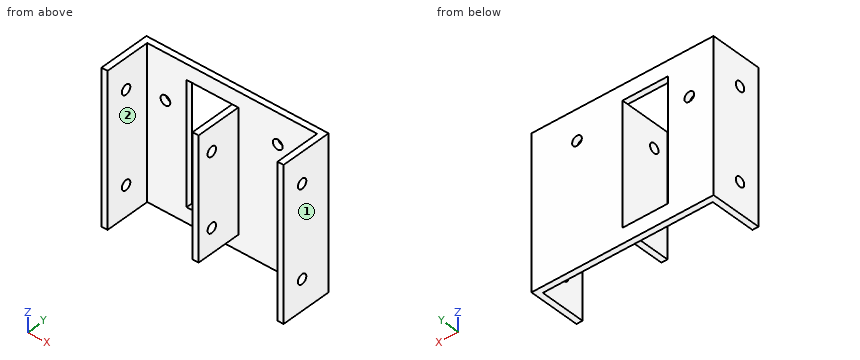
from build123d import *

# Parameters (mm, degrees)
BOSS_EXTRUDE1_DEPTH = 50
SKETCH2_R           = 1.6
CUT_EXTRUDE1_DEPTH  = 80.931220434
SKETCH3_W           = 2
SKETCH3_H           = 40
BOSS_EXTRUDE2_DEPTH = 17
SKETCH5_R           = 1.6
CUT_EXTRUDE3_DEPTH  = 2
SKETCH6_R           = 1.6
CUT_EXTRUDE4_DEPTH  = 80.931220434
SKETCH7_W           = 15
SKETCH7_H           = 40
CUT_EXTRUDE5_DEPTH  = 2


with BuildPart() as part:
    # Sketch1 → Boss-Extrude1 (new body)
    with BuildSketch(Plane.XY):
        Polygon((0, 0), (0, 17), (60, 17), (60, 0), (58, 0), (58, 15), (2, 15), (2, 0), align=None)
    extrude(amount=BOSS_EXTRUDE1_DEPTH)

    # Sketch2 → Cut-Extrude1 (cut, through all)
    with BuildSketch(Plane(origin=(60, 0, 0), x_dir=(0, 0, -1), z_dir=(1, 0, 0))):
        with Locations(Location((-40, 7, 0), (0, 0, 90))):
            Circle(SKETCH2_R)
        with Locations(Location((-10, 7, 0), (0, 0, 180))):
            Circle(SKETCH2_R)
    extrude(amount=-CUT_EXTRUDE1_DEPTH, mode=Mode.SUBTRACT)

    # Sketch3 → Boss-Extrude2 (add)
    with BuildSketch(Plane(origin=(0, 17, 0), x_dir=(1, 0, 0), z_dir=(0, 1, 0))):
        with Locations((31, -25)):
            Rectangle(SKETCH3_W, SKETCH3_H)
    extrude(amount=-BOSS_EXTRUDE2_DEPTH)

    # Sketch5 → Cut-Extrude3 (cut)
    with BuildSketch(Plane(origin=(32, 0, 0), x_dir=(0, 0, -1), z_dir=(1, 0, 0))):
        with Locations((-37, 5)):
            Circle(SKETCH5_R)
        with Locations(Location((-13, 5, 0), (0, 0, 180))):
            Circle(SKETCH5_R)
    extrude(amount=-CUT_EXTRUDE3_DEPTH, mode=Mode.SUBTRACT)

    # Sketch6 → Cut-Extrude4 (cut, through all)
    with BuildSketch(Plane(origin=(0, 17, 0), x_dir=(1, 0, 0), z_dir=(0, 1, 0))):
        with Locations(Location((45, -40, 0), (0, 0, 270))):
            Circle(SKETCH6_R)
        with Locations(Location((8, -35, 0), (0, 0, 270))):
            Circle(SKETCH6_R)
    extrude(amount=-CUT_EXTRUDE4_DEPTH, mode=Mode.SUBTRACT)

    # Sketch7 → Cut-Extrude5 (cut)
    with BuildSketch(Plane.XZ.offset(-15)):
        with Locations((22.5, 25)):
            Rectangle(SKETCH7_W, SKETCH7_H)
    extrude(amount=-CUT_EXTRUDE5_DEPTH, mode=Mode.SUBTRACT)


solid = part.part
Model file for the job. Use its own axes, mm. Face numbers are marked on the shaded views. A direction names the side the tool comes from. Round coordinates to 2 decimals unless told otherwise and drop trailing zeros. Order: outer loops, then holes, each group sorted by start corner. A loop starts at its lowest first (then second) coordinate and runs counter-clockwise, first axis right, second up.
(1) Band-saw the part on C-C (z = 16.5). List the corners of the cut face in (x, y), then the cut area to 3 significant figures.
(2) Band-saw the part on B-B (z = 10). List the corners of the cut face in (x, y), then the cut area to 3 significant figures.
(3) Drill centre lines: line 1 (X direction, y = 6.25, z = 43); line 2 (Z direction, x = 59.3, y = 7); line 3 (X direction, y = 9, z = 46). Where is each one in solid material? Low to high.
(4) Pin check, flat tips, straight feed: pin 1 (0.6 mm diameter, centred on x = 31.5, y = 6, fed in from +Z); pin 2 (2 mm diameter, centred on x = 31.5, y = 8.5, fed in from -Z); pin 3 (2.5 mm diameter, centred on y = 7, z = 40, fed in from -X). Stop position of each tip, or through.
(5) 3-axis set-ups, long thin cutter, end or side, ignore diameter. For the marked faces 1 and 2: which of +Z, -Z, +X, -X, +Y, -Y reach the whole face in a straight line?
(6) Band-saw the part on A-A (x = 8). List the corners of the cut face in (y, z), then the cut area to 3 significant figures.
(7) Band-saw the part on D-D (y = 4.25). List the corners of the cut face in (x, z).
Verdict:
1. outline: (0, 0) - (2, 0) - (2, 15) - (15, 15) - (15, 17) - (0, 17) - close; (30, 0) - (32, 0) - (32, 15) - (58, 15) - (58, 0) - (60, 0) - (60, 17) - (30, 17) - close
1. area: 180 mm2
2. outline: (0, 0) - (2, 0) - (2, 5.4) - (0, 5.4) - close; (0, 8.6) - (2, 8.6) - (2, 15) - (15, 15) - (15, 17) - (0, 17) - close; (30, 0) - (32, 0) - (32, 15) - (58, 15) - (58, 8.6) - (60, 8.6) - (60, 17) - (30, 17) - close; (58, 0) - (60, 0) - (60, 5.4) - (58, 5.4) - close
2. area: 167 mm2
3. line 1: x = 0 to 2, 30 to 32, 58 to 60
3. line 2: z = 0 to 8.4, 11.6 to 38.4, 41.6 to 50
3. line 3: x = 0 to 2, 58 to 60
4. pin 1: stops at z = 45
4. pin 2: stops at z = 5
4. pin 3: stops at x = 30
5. face 1: +Z, -Z, +X, +Y, -Y
5. face 2: +Z, -Z, -Y
6. outline: (15, 0) - (17, 0) - (17, 33.4) - (15, 33.4) - close; (15, 36.6) - (17, 36.6) - (17, 50) - (15, 50) - close
6. area: 93.6 mm2
7. outline: (0, 0) - (2, 0) - (2, 50) - (0, 50) - close; (30, 5) - (32, 5) - (32, 11.59) - (30, 11.59) - close; (30, 14.41) - (32, 14.41) - (32, 35.59) - (30, 35.59) - close; (30, 38.41) - (32, 38.41) - (32, 45) - (30, 45) - close; (58, 0) - (60, 0) - (60, 50) - (58, 50) - close
